Input: dimensioned drawing with shaded views. Units: mm. Origin: part minimum x, y, z. Round coordinates to 2 decimals unless told otherwise and drop trailing zeros. Order: outer loops, then holes, each group sorted by start corner. A loop starts at its lowest first (then second) coordinate and runs counter-clockwise, first axis right, second up. Notation, with made-up numbers: M -16.75,46 L -2.75,46 A17 ccw -2.75,63 Z; hole C -6,16 d8. An arc over 180 degrees is marked long. One line per question, with ' | ' between items.
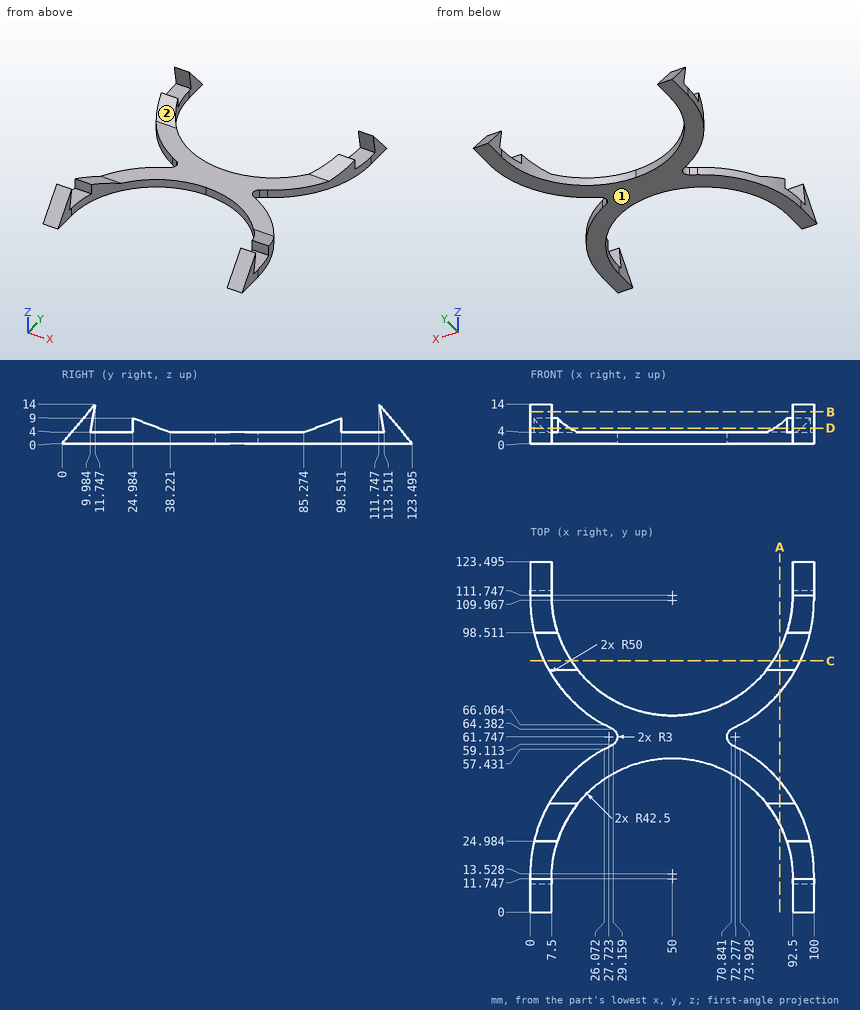
Item 1: Section query B-B, the plane z = 11.25. Return loops of the section in (x, y) (1 decimal).
Report:
outline: M 0,9.4 L 7.5,9.4 L 7.5,11.3 L 0,11.3 Z; M 0,112.2 L 7.5,112.2 L 7.5,114.1 L 0,114.1 Z; M 92.5,9.4 L 100,9.4 L 100,11.3 L 92.5,11.3 Z; M 92.5,112.2 L 100,112.2 L 100,114.1 L 92.5,114.1 Z
Item 2: Line query: line 1 along Y through (x, z) = (81.5, 2.25) (1 decimal); line 2 along X through (y, z) = (114, 1.25); line 3 along X through (y, z) = (15.5, 1.5) (1 decimal). Output: solid intervals per line, ascending. Write a range as from..to.
Report:
line 1: 40.3..52.4, 71.1..83.2 | line 2: 0..7.5, 92.5..100 | line 3: 0..7.7, 92.3..100
Item 3: Section query D-D, the plane z = 5.5. Give the number of separate pieces and of enclosed holes in the cut face.
Report:
separate pieces: 8 | enclosed holes: 0
Item 4: First-contact query: pin 1 (7.5 mm diameter, centred on x = 97.5, y = 106, fed in from +Z); pin 2 (4 mm diameter, centred on x = 4.5, z = 7, fed in from +Y); pin 3 (1 mm diameter, centred on y = 17, z = 3.5, fed in from -X). Flat tips, straight axial feed; report the tip coordinate or a pass-through.
Report:
pin 1: z = 4 | pin 2: y = 119.3 | pin 3: x = 0.09
Item 5: Mould query, pull axis Y, two halves, no side actions, for the marked faces 1 and 2. Classes: +Y half, -Y half, draft (parallel to the pull), parting line (faces both ways), or undercut.
Report:
face 1: draft | face 2: undercut
Item 6: Section query A-A, the plane x = 88. Return loops of the section in (y, z) (1 decimal).
Report:
outline: M 30.8,0 L 46,0 L 46,4 L 38.2,4 L 30.8,6.8 Z; M 77.5,0 L 92.7,0 L 92.7,6.8 L 85.3,4 L 77.5,4 Z
Item 7: Section query C-C, the plane y = 88.5. Return loops of the section in (x, z).
Report:
outline: M 4.84,0 L 14.42,0 L 14.42,5.22 L 4.84,5.22 Z; M 85.58,0 L 95.16,0 L 95.16,5.22 L 85.58,5.22 Z
